```python
from build123d import *

# Parameters (mm, degrees)
F1_DEPTH = 19
F3_DEPTH = 180.001
F5_D     = 5.5
F6_R     = 7.7
F6_R_2   = 8.5
F7_DEPTH = 19.001
F9_R     = 17
F9_R_2   = 13
F12_R    = 14
F12_R_2  = 8.5


with BuildPart() as f1:
    # F0 (on Front) → F1 (new body)
    with BuildSketch(Plane.XZ):
        with BuildLine():
            Line((0, 55), (0, 0))
            Line((0, 0), (180, 0))
            Line((180, 0), (180, 55))
            ThreePointArc((180, 55), (90, 112.4), (0, 55))
        make_face()
    extrude(amount=F1_DEPTH)

    # F2 (on face) → F3 (cut, through all)
    with BuildSketch(Plane.YZ.offset(180)):
        Polygon((0, 112.4), (-9, 0), (0, 0), align=None)
    extrude(amount=-F3_DEPTH, mode=Mode.SUBTRACT)

    # F5 (through all)
    with Locations(Plane.XZ.offset(19)):
        with Locations((32.5, 30), (147.5, 30)):
            Hole(F5_D / 2)

    # F6 (on face) → F7 (cut, through all)
    with BuildSketch(Plane.XZ.offset(19)):
        with Locations((90, 83.3)):
            Circle(F6_R)
        with Locations((131.35, 81)):
            Circle(F6_R_2)
        with Locations((48.65, 81)):
            Circle(F6_R_2)
    extrude(amount=-F7_DEPTH, mode=Mode.SUBTRACT)

    # F9 (on offset) → F10 (join, up to the next surface of F1)
    with BuildSketch(Plane.XZ.offset(-5)):
        with Locations((90, 83.3)):
            Circle(F9_R)
        with Locations((90, 83.3)):
            Circle(F9_R_2, mode=Mode.SUBTRACT)
    extrude(until=Until.NEXT)

    # F12 (on offset) → F13 (join, up to the next surface of F1)
    with BuildSketch(Plane.XZ.offset(-1)):
        with Locations((131.35, 81)):
            Circle(F12_R)
        with Locations((131.35, 81)):
            Circle(F12_R_2, mode=Mode.SUBTRACT)
        with Locations((48.65, 81)):
            Circle(F12_R)
        with Locations((48.65, 81)):
            Circle(F12_R_2, mode=Mode.SUBTRACT)
    extrude(until=Until.NEXT)


solid = f1.part
```
The model under review builds one solid part; all positions refer to its coordinate system, in mm. A direction names the side the tool comes from. Round coordinates to 2 decimals unless told otherwise and drop trailing zeros. Write each loop counter-clockwise with the first axis right and the second up, starting at its lowest first coordinate (ties: lowest second). Pieces come first, ordered by that corner, then holes.
(1) Machinability: for faces 1 (the flat face through (55, 1, 75)), 2 (the flat face through (140, 1, 81)), 3 (the cylindrical face through (87.18, 0.86, 70.61)), which of the approach directions +Z, -Z, +X, -X, +Y, -Y give a long, thin tool a straight path to every point of the face, cutting with its end or side? Answer none if there is none.
(2) We need section C-C on y = -15.25. Give the boundary of the cut face in (x, z), and give its area (3 significant figures).
(3) We need section D-D on z = 30. Give the boundary of the cut face in (x, y), and give its area (3 significant figures).
(4) We need section A-A on z = 79. Give the number of separate pieces and of enclosed holes in the cut face, and give its area (3 significant figures).
(5) Wall thickness on L1, parallel to X at y = -11.25, z = 30; L2, parallel to X at y = -15.25, z = 86; L3, parallel to X at y = -11.75, z = 81: over which ranges is each line inside the solid? List them lowest first.
(6) Insertion check: pin 1 (12 mm diameter, centred on y = -15, z = 68, fed in from +X); pin 2 (10 mm diameter, centred on x = 64.5, y = -1, fed in from +Z); pin 3 (8 mm diameter, centred on x = 106.5, z = 22.5, fed in from +Y); pin 4 (19.5 mm diameter, centred on x = 131.35, z = 81, fed in from -Y). Each pin has a flat end and moves straight along its axis. Give the tip position at first contact, or say it passes through.
(7) We need section B-B on x = 31.5. Give the boundary of the cut face in (y, z), and give its area (3 significant figures).
Findings below:
1. face 1: +Z, -Z, -X, +Y
1. face 2: +Z, -Z, +X, +Y
1. face 3: +Y
2. outline: (0, 0) - (180, 0) - (180, 55) arc R99.26 ccw to (0, 55) - close; hole circle Ø5.5 at (32.5, 30); hole circle Ø17 at (48.65, 81); hole circle Ø15.4 at (90, 83.3); hole circle Ø17 at (131.35, 81); hole circle Ø5.5 at (147.5, 30)
2. area: 16,600 mm2
3. outline: (0, -19) - (29.75, -19) - (29.75, -6.6) - (0, -6.6) - close; (35.25, -19) - (144.75, -19) - (144.75, -6.6) - (35.25, -6.6) - close; (150.25, -19) - (180, -19) - (180, -6.6) - (150.25, -6.6) - close
3. area: 2,100 mm2
4. separate pieces: 4
4. enclosed holes: 0
4. area: 1,820 mm2
5. L1: x = 0 to 29.75, 35.25 to 144.75, 150.25 to 180
5. L2: x = 22.59 to 41.78, 55.52 to 82.79, 97.21 to 124.48, 138.22 to 157.41
5. L3: x = 17.56 to 40.15, 57.15 to 82.65, 97.35 to 122.85, 139.85 to 162.44
6. pin 1: stops at x = 176.4
6. pin 2: stops at z = 110.26
6. pin 3: stops at y = -6.88
6. pin 4: stops at y = -19
7. outline: (-19, 0) - (-9, 0) - (-6.8, 27.44) - (-19, 27.44) - close; (-19, 32.56) - (-6.39, 32.56) - (-1.53, 93.33) - (-19, 93.33) - close
7. area: 1,220 mm2
